Check sheet for the modelled part. Datum: model origin and axes. Units: mm. A direction names the side the tool comes from. Coordinates: 2 decimals unless noted, no trailing zeros. Loops run counter-clockwise (first coordinate to the right, second up) from the corner with the lowest first, then second, coordinate; pieces in that order, holes last. Notation, with made-up numbers: (-7, 80.5) - (41, 80.5) arc R7 ccw to (41, 88.5) - close; hole circle Ø5 at (-31.5, 6.5). An arc over 180 degrees is marked (long way). Use a Markdown table: item, result. Add a question column.
1) Sectioned sample at C-C, the plane y = 15.5. Enter the section's corners in (x, z), then the cut area to 3 significant figures.
2) Sectioned sample at B-B, the plane y = -3. Enter the section's corners in (x, z), then the cut area to 3 significant figures.
3) Draft check along Z on faces 4 (the flat face through (-10, 26.802, -74)), 5 (the cylindrical face through (-5.31, -25.4, -73.95)), 6 (the flat face through (-6, 32, -124.396)), 7 (the flat face through (-1, 3, 0)). Enter one of: pulls with the +Z half, pulls with the -Z half, needs draft (parallel to the pull), parting line crosses it, or undercut.
4) Sectioned sample at A-A, the plane z = -67.5. Enter the section's corners in (x, y) (3 decimals).
5) Thickness scan on line 1 (Z direction, x = -1.75, y = 28.5); line 2 (X direction, y = 10, z = -50.5); line 3 (Y direction, x = -8.25, z = -78.5). Record the ranges inside material, lowest first.
6) Go/stop test with flat-tipped pins: P1, Ø3, axis at x = -8, z = -35.5, coming from the -Y side; P2, Ø1.5, axis at x = -10.5, z = -74, coming from the +Y side; P3, Ø10, axis at y = -1, z = -123.5, coming from the -X side. Record where each tip stops, or that it passes through.
7) Tool access check on faces 1 (the flat face through (-10, -26.802, -74)), 2 (the cylindrical face through (-2.9, -18.2, -76)), 3 (the flat face through (-2, 26.802, -74)). Record the directions out of +Z, -Z, +X, -X, +Y, -Y that give a thin tool (end or side, any length) a straight path to the whole face; none if there is none.
from build123d import *

# Parameters (mm, degrees)
CROQUIS1_R              = 3.175
SALIENTE_EXTRUIR1_DEPTH = 150
REDONDEO1_R             = 10
CROQUIS3_W              = 98.791812306
CROQUIS3_H              = 18.145434914
CORTAR_EXTRUIR2_DEPTH   = 155.383451186


with BuildPart() as part:
    # Croquis1 → Saliente-Extruir1 (new body)
    with BuildSketch(Plane.XY):
        with BuildLine():
            Line((-1.6, 19.056228096), (-8.98691391, 23.296314259))
            ThreePointArc((-8.98691391, 23.296314259), (-9.006535925, 33.69237342), (0, 28.5))
            Line((0, 28.5), (0, -28.5))
            ThreePointArc((0, -28.5), (-9.006535925, -33.69237342), (-8.98691391, -23.296314259))
            Line((-8.98691391, -23.296314259), (-1.6, -19.056228096))
            Line((-1.6, -19.056228096), (-1.6, 19.056228096))
        make_face()
        with Locations((-6, 28.5)):
            Circle(CROQUIS1_R, mode=Mode.SUBTRACT)
        with Locations(Location((-6, -28.5, 0), (0, 0, 180))):
            Circle(CROQUIS1_R, mode=Mode.SUBTRACT)
    extrude(amount=-SALIENTE_EXTRUIR1_DEPTH)

    # Redondeo1
    redondeo1_edges = [part.edges().sort_by_distance(p)[0] for p in [
        (-1.6, -19.056228096, -75),
        (-1.6, 19.056228096, -75),
    ]]
    fillet(redondeo1_edges, radius=REDONDEO1_R)

    # Croquis3 → Cortar-Extruir2 (cut, through all)
    with BuildSketch(Plane(origin=(0, 0, 0), x_dir=(0, 0, -1), z_dir=(1, 0, 0))):
        with Locations((75, 35.875128035)):
            Rectangle(CROQUIS3_W, CROQUIS3_H)
        with Locations((75, -35.875128035)):
            Rectangle(CROQUIS3_W, CROQUIS3_H)
    extrude(amount=-CORTAR_EXTRUIR2_DEPTH, mode=Mode.SUBTRACT)


solid = part.part
Solved:
| question | item | result |
|---|---|---|
| 1 | outline | (-1.85, -150) - (0, -150) - (0, 0) - (-1.85, 0) - close |
| 1 | area | 278 mm2 |
| 2 | outline | (-1.6, -150) - (0, -150) - (0, 0) - (-1.6, 0) - close |
| 2 | area | 240 mm2 |
| 3 | face 4 | undercut |
| 3 | face 5 | needs draft |
| 3 | face 6 | undercut |
| 3 | face 7 | pulls with the +Z half |
| 4 | outline | (-11.755, -26.802) - (-8.683, -26.802) arc R3.175 cw to (-3.317, -26.802) - (0, -26.802) - (0, 26.802) - (-3.317, 26.802) arc R3.175 cw to (-8.683, 26.802) - (-11.755, 26.802) arc R6 ccw to (-8.987, 23.296) - (-6.622, 21.939) arc R10 cw to (-1.6, 13.266) - (-1.6, -13.266) arc R10 cw to (-6.622, -21.939) - (-8.987, -23.296) arc R6 ccw to start |
| 5 | line 1 | z = -150 to -124.4, -25.6 to 0 |
| 5 | line 2 | x = -1.6 to 0 |
| 5 | line 3 | y = -26.26 to -22.87, 22.87 to 26.26 |
| 6 | P1 | stops at y = -26.8 |
| 6 | P2 | stops at y = 26.8 |
| 6 | P3 | stops at x = -1.6 |
| 7 | face 1 | +X, -X, -Y |
| 7 | face 2 | +Z, -Z, -X |
| 7 | face 3 | +X, -X, +Y |
